from build123d import *

# Parameters (mm, degrees)
SKETCH_1_R          = 15
SKETCH_1_R_2        = 4
EXTRUDE_1_DEPTH     = 35
SKETCH_2_R          = 7.5
CUT_EXTRUDE_1_DEPTH = 15
SKETCH_3_R          = 2
CUT_EXTRUDE_2_DEPTH = 6
SKETCH_4_R          = 3.5
CUT_EXTRUDE_3_DEPTH = 10
CUT_EXTRUDE_START   = -2
SKETCH_5_R          = 15
SKETCH_5_R_2        = 12
CUT_EXTRUDE_4_DEPTH = 2
SKETCH_6_R          = 2
CUT_EXTRUDE_5_DEPTH = 20
CHAMFER_1_SIZE      = 0.5


with BuildPart() as part:
    # 草图1 → 凸台-拉伸1 (new body)
    with BuildSketch(Plane.XY):
        Circle(SKETCH_1_R)
        Circle(SKETCH_1_R_2, mode=Mode.SUBTRACT)
    extrude(amount=EXTRUDE_1_DEPTH)

    # 草图2 → 切除-拉伸1 (cut)
    with BuildSketch(Plane.XY.offset(35)):
        Circle(SKETCH_2_R)
    extrude(amount=-CUT_EXTRUDE_1_DEPTH, mode=Mode.SUBTRACT)

    # 草图3 → 切除-拉伸2 (cut, symmetric)
    with BuildSketch(Plane(origin=(0, 0, 0), x_dir=(0, 0, -1), z_dir=(1, 0, 0))):
        with Locations((-8.856511141, 10.195845598)):
            Circle(SKETCH_3_R)
    extrude(amount=CUT_EXTRUDE_2_DEPTH, both=True, mode=Mode.SUBTRACT)

    # 草图4 → 切除-拉伸3 (cut)
    with BuildSketch(Plane.ZY.offset(14)):
        with Locations((8.856511141, 10.195845598)):
            Circle(SKETCH_4_R)
    extrude(amount=-CUT_EXTRUDE_3_DEPTH, mode=Mode.SUBTRACT)

    # 草图5 → 切除-拉伸4 (cut)
    with BuildSketch(Plane.XY.offset(20).offset(CUT_EXTRUDE_START)):
        Circle(SKETCH_5_R)
        Circle(SKETCH_5_R_2, mode=Mode.SUBTRACT)
    extrude(amount=CUT_EXTRUDE_4_DEPTH, mode=Mode.SUBTRACT)

    # 草图6 → 切除-拉伸5 (cut, symmetric)
    with BuildSketch(Plane(origin=(0, 0, 0), x_dir=(0, 0, -1), z_dir=(1, 0, 0))):
        with Locations((-27.877925761, -10.249978731)):
            Circle(SKETCH_6_R)
    extrude(amount=CUT_EXTRUDE_5_DEPTH, both=True, mode=Mode.SUBTRACT)

    # 倒角1
    chamfer_1_edges = [part.edges().sort_by_distance(p)[0] for p in [
        (-15, 0, 0),
        (-15, 0, 35),
    ]]
    chamfer(chamfer_1_edges, length=CHAMFER_1_SIZE)


solid = part.part
Build history of the part. All positions in model axes, mm. A direction names the side the tool comes from. Round coordinates to 2 decimals unless told otherwise and drop trailing zeros. Write each loop counter-clockwise with the first axis right and the second up, starting at its lowest first coordinate (ties: lowest second). Pieces come first, ordered by that corner, then holes. Notation, with made-up numbers: M 7.25,39.5 L 48.25,39.5 A23 cw 48.25,58.5 Z; hole C -27,12.5 d11. An arc over 180 degrees is marked long. Answer in a Markdown table with one row per item.
1. Probe L1, parallel to Z at x = -0.5, y = 10; L2, parallel to Y at x = 0, z = 31; L3, parallel to Y at x = 0, z = 14. List the from-to ranges inside material, lowest first. Write a range as [from, to].
Geometry check:
| item | result |
|---|---|
| L1 | [0, 6.87], [10.85, 35] |
| L2 | [-15, -7.5], [7.5, 15] |
| L3 | [-15, -4], [4, 15] |
2. Saw through at B-B (x = 0). List the corners of the cut face in (y, z), and give its area (3 significant figures).
Geometry check:
| item | result |
|---|---|
| outline | M -15,0.5 L -14.5,0 L -4,0 L -4,20 L -7.5,20 L -7.5,35 L -14.5,35 L -15,34.5 L -15,20 L -12,20 L -12,18 L -15,18 Z; M 4,0 L 14.5,0 L 15,0.5 L 15,18 L 12,18 L 12,20 L 15,20 L 15,34.5 L 14.5,35 L 7.5,35 L 7.5,20 L 4,20 Z; hole C -10.25,27.88 d4; hole C 10.2,8.86 d4 |
| area | 627 mm2 |
3. Flat gauge pins, fed straight in: P1, Ø4, axis at x = -6.5, z = 19.5, coming from the -Y side; P2, Ø3.5, axis at y = 10.2, z = 8.86, coming from the -X side; P3, Ø7.5, axis at x = 2.5, y = -2, coming from the +Z side. Where does each tip first touch, or does it go through?
Geometry check:
| item | result |
|---|---|
| P1 | y = -14.29 |
| P2 | x = 6 |
| P3 | z = 20 |
4. Which spindle directions (+Z, -Z, +X, -X, +Y, -Y) get a long thin tool onto all of the face, cutting with end or side? Do faces 1 (the face through (-7.73, 6.78, 8.1)), 2 (the face through (3, -3, 0)), 3 (the face through (3, -3, 20)), 4 (the face through (-11.99, 0.53, 18.99)). Say none if no direction does.
Geometry check:
| item | result |
|---|---|
| face 1 | -X |
| face 2 | -Z, +X, -X, +Y, -Y |
| face 3 | +Z |
| face 4 | none |
5. Saw through at D-D (z = 14). List the corners of the cut face in (x, y), and give its area (3 significant figures).
Geometry check:
| item | result |
|---|---|
| outline | C 0,0 d30; hole C 0,0 d8 |
| area | 657 mm2 |
6. Saw through at A-A (y = 0). List the corners of the cut face in (x, z).
Geometry check:
| item | result |
|---|---|
| outline | M -15,0.5 L -14.5,0 L -4,0 L -4,20 L -7.5,20 L -7.5,35 L -14.5,35 L -15,34.5 L -15,20 L -12,20 L -12,18 L -15,18 Z; M 4,0 L 14.5,0 L 15,0.5 L 15,18 L 12,18 L 12,20 L 15,20 L 15,34.5 L 14.5,35 L 7.5,35 L 7.5,20 L 4,20 Z |
7. Saw through at C-C (z = 19). List the corners of the cut face in (x, y), and give its area (3 significant figures).
Geometry check:
| item | result |
|---|---|
| outline | C 0,0 d24; hole C 0,0 d8 |
| area | 402 mm2 |
8. Mould opens along X. For faces 5 (the face through (8.06, 12.65, 27.15)), 6 (the face through (6, 10, 9)), 7 (the face through (-0.867, -3.905, 9.86)) say: +X half, -X half, draft (parallel to the pull), parting line (faces both ways), or undercut.
Geometry check:
| item | result |
|---|---|
| face 5 | parting line |
| face 6 | -X half |
| face 7 | undercut |
